Autodesk Inventor part; units mm, degrees
ref_plane "YZ Plane" through (0, 0, 0) normal (1, 0, 0) x (0, 1, 0)
ref_plane "XZ Plane" through (0, 0, 0) normal (0, 1, 0) x (-1, 0, 0)
ref_plane "XY Plane" through (0, 0, 0) normal (0, 0, 1) x (1, 0, 0)
sketch "Sketch1" plane through (0, 0, 0) normal (0, 1, 0) x (-1, 0, 0)
  line L0 (0, 0) -> (-66.5, 0)
  line L1 (-66.5, 0) -> (-66.5, -52.5)
  line L2 (-66.5, -52.5) -> (0, -52.5)
  line L3 (0, -52.5) -> (0, 0)
  dimension "d0" = 52.5
  dimension "d1" = 66.5
extrude "Extrusion1" add sketch "Sketch1" along normal blind 3
sketch "Sketch2" plane through (0, 3, 0) normal (0, 1, 0) x (1, 0, 0)
  line L0 (0, 0) -> (66.5, 0)
  line L1 (66.5, 0) -> (66.5, 52.5)
  line L2 (33.31, 0) -> (42.31, 0)
  line L3 (42.31, 0) -> (42.31, 3)
  line L4 (42.31, 3) -> (33.31, 3)
  line L5 (33.31, 3) -> (33.31, 0)
  point P0 (37.81, 3)
  dimension "d5" = 9
  dimension "d6" = 3
  dimension "d7" = 28.69
extrude "Extrusion2" add sketch "Sketch2" along normal blind 0.4
sketch "Sketch4" plane through (0, 0, 0) normal (0, -1, 0) x (1, 0, 0)
  line L0 (66.5, -52.5) -> (0, -52.5)
  line L1 (66.5, 0) -> (66.5, -52.5)
  line L2 (61.5, -47.5) -> (5, -47.5) construction
  line L3 (5, -47.5) -> (5, -5) construction
  line L4 (5, -5) -> (61.5, -5) construction
  line L5 (61.5, -5) -> (61.5, -47.5) construction
  point P0 (33.25, -47.5)
  point P1 (33.25, -52.5)
  point P2 (61.5, -26.25)
  point P3 (66.5, -26.25)
  dimension "d12" = 56.5
  dimension "d13" = 42.5
hole "Hole1" at (61.5, 0, -47.5) at (5, 0, -47.5) at (5, 0, -5) at (61.5, 0, -5) direction (0, 1, 0) diameter 3 end through all countersink diameter 7 countersink angle 90
sketch "Sketch5" plane through (0, 3, 0) normal (0, 1, 0) x (1, 0, 0)
  line L0 (66.5, 52.5) -> (0, 52.5)
  line L1 (0, 52.5) -> (0, 0)
  line L2 (56.11, 3.39) -> (10.39, 3.39) construction
  line L3 (10.39, 3.39) -> (10.39, 49.11) construction
  line L4 (10.39, 49.11) -> (56.11, 49.11) construction
  line L5 (56.11, 49.11) -> (56.11, 3.39) construction
  point P0 (33.25, 49.11)
  point P1 (33.25, 52.5)
  point P2 (10.39, 26.25)
  point P3 (0, 26.25)
  point P4 (33.25, 44.11)
  dimension "d21" = 45.72
  dimension "d22" = 5
  dimension "d23" = 22.86
hole "Hole2" at (33.25, 3, -44.11) direction (0, -1, 0) diameter 3 end through all countersink diameter 8 countersink angle 90
fillet "Fillet1" radius 6 4 edges at (0, 1.5, -52.5) (66.5, 1.5, -52.5) (66.5, 1.5, 0) (0, 1.5, 0)
properties part number "top"
Read the model definition and answer for the solid it produces. Units are mm, in the model's axes. Coordinates: 2 decimals unless noted, no trailing zeros. Order: outer loops, then holes, each group sorted by start corner. A loop starts at its lowest first (then second) coordinate and runs counter-clockwise, first axis right, second up. Notation, with made-up numbers: M 20,2 L 41,2 A14 ccw 41,6 Z; hole C 11.25,88.25 d3. An arc over 180 degrees is marked long. Put each result on its own line as item: value. Start each with the question number.
Item 1: Given pin 1 Ø5 at (x, z) = (61.5, -5) entering from -Y; pin 2 Ø2 at (y, z) = (0.5, -27) entering from -X; pin 3 Ø2.5 at (x, z) = (33.25, -44.11) entering from +Y; pin 4 Ø4 at (x, z) = (5, -47.5) entering from +Y, each flat-ended and moving along its own axis, determine where each tip first touches the part or whether it passes through.
Item 2: Consider probe 1 along Z at (x, y) = (33.25, 0.2); probe 2 along X at (y, z) = (2.65, -5); probe 3 along Z at (x, y) = (61.5, 2.2). Determine where each line is inside the solid, lowest interval first. Write a range as [from, to].
Item 3: Section C-C, the plane z = -26 is taken. Determine the outline of the cut face in (x, y).
Item 4: Section D-D, the plane x = 20.5 is taken. Determine the outline of the cut face in (y, z).
Item 5: Section B-B, the plane x = 38.5 is taken. Determine the outline of the cut face in (y, z).
Item 6: The mould has two halves that part along Z. Classify faces 1 (the face through (59.91, 1.87, -4.65)), 2 (the face through (33, 2, 0)), 3 (the face through (38, 3.4, -2)): +Z half, -Z half, draft (parallel to the pull), parting line (faces both ways), or undercut.
Item 7: Section A-A, the plane z = -5 is taken. Determine the outline of the cut face in (x, y).
Computed:
1. pin 1: stops at y = 1
1. pin 2: stops at x = 0
1. pin 3: passes through
1. pin 4: stops at y = 3
2. probe 1: z = [-52.5, -45.61], [-42.61, 0]
2. probe 2: x = [0.08, 3.5], [6.5, 60], [63, 66.42]
2. probe 3: z = [-52.42, -49], [-46, -6.5], [-3.5, -0.08]
3. outline: M 0,0 L 66.5,0 L 66.5,3 L 0,3 Z
4. outline: M 0,-52.5 L 3,-52.5 L 3,0 L 0,0 Z
5. outline: M 0,-52.5 L 3,-52.5 L 3,-3 L 3.4,-3 L 3.4,0 L 0,0 Z
6. face 1: undercut
6. face 2: +Z half
6. face 3: draft
7. outline: M 0.08,0 L 1.5,0 L 3.5,2 L 3.5,3 L 0.08,3 Z; M 6.5,2 L 8.5,0 L 58,0 L 60,2 L 60,3 L 6.5,3 Z; M 63,2 L 65,0 L 66.42,0 L 66.42,3 L 63,3 Z
